```python
from build123d import *

# Parameters (mm, degrees)
F0_R     = 70
F1_DEPTH = 1
F3_R     = 1.99999


# Not quite as in the source:
# - a fillet or chamfer is up to 0.001 mm smaller than in the source, because OpenCascade refuses the exact size
# - a feature of the source that left no trace in its solid (it failed there, or was rolled back) is left out


with BuildPart() as f1:
    # F0 (on Front) → F1 (new body, symmetric)
    with BuildSketch(Plane.XZ):
        Circle(F0_R)
        Polygon((-30.855941539, 30.855941539), (-11.294058461, 42.15), (11.294058461, 42.15), (30.855941539, 30.855941539), (42.15, 11.294058461), (42.15, -11.294058461), (30.855941539, -30.855941539), (11.294058461, -42.15), (-11.294058461, -42.15), (-30.855941539, -30.855941539), (-42.15, -11.294058461), (-42.15, 11.294058461), align=None, mode=Mode.SUBTRACT)
    extrude(amount=F1_DEPTH, both=True)

    # F3 (radius 2 in the source; OpenCascade refuses exactly that, so slightly less here)
    f3_edges = [f1.edges().sort_by_distance(p)[0] for p in [
        (-21.075, -1, 36.502971),
        (0, -1, 42.15),
        (21.075, -1, 36.502971),
        (36.502971, -1, 21.075),
        (42.15, -1, 0),
        (36.502971, -1, -21.075),
        (21.075, -1, -36.502971),
        (0, -1, -42.15),
        (-21.075, -1, -36.502971),
        (-36.502971, -1, -21.075),
        (-42.15, -1, 0),
        (-36.502971, -1, 21.075),
    ]]
    fillet(f3_edges, radius=F3_R)


solid = f1.part
```
Geometry: final body of the model. Coordinates: model frame, mm. Round coordinates to 2 decimals unless told otherwise and drop trailing zeros. Order: outer loops, then holes, each group sorted by start corner. A loop starts at its lowest first (then second) coordinate and runs counter-clockwise, first axis right, second up. Notation, with made-up numbers: (83.25, 32) -> (106.25, 32) arc R7 ccw to (106.25, 42) -> close; hole circle Ø6 at (-27, -18). An arc over 180 degrees is marked (long way). Use one line per item in the form item = value. Start each with the question number.
1. Cut plane C-C (y = -0.5). Return the cut outline in (x, z).
2. Pin query (flat end, axial travel): pin 1 Ø8 at (x, z) = (-31, 29) entering from -Y; pin 2 Ø1 at (y, z) = (0, -44) entering from +X; pin 3 Ø1 at (y, z) = (-0.5, 32) entering from +X. Return the tip coordinate at first contact, or that it passes through.
3. Draft query along X for faces 1 (the face through (-21.23, -0.43, 37.11)), 2 (the face through (-21.52, -0.43, -36.94)), 3 (the face through (30, 1, 32)), 4 (the face through (-55.55, -0.014, -42.594)). Return one class per face: pulls with the +X half, pulls with the -X half, needs draft (parallel to the pull), parting line crosses it, or undercut.
4. Line query: probe 1 along X at (y, z) = (0.3, 3); probe 2 along X at (y, z) = (-0.35, -2.5); probe 3 along Z at (x, y) = (4, -0.15). Output: solid intervals per line, ascending.
5. Cut plane D-D (x = -47). Return the cut outline in (y, z), then the cut area to 4 significant figures.
Solution:
q1.outline = circle Ø140 at (0, 0); hole (-42.83, -11.48) -> (-31.35, -31.35) -> (-11.48, -42.83) -> (11.48, -42.83) -> (31.35, -31.35) -> (42.83, -11.48) -> (42.83, 11.48) -> (31.35, 31.35) -> (11.48, 42.83) -> (-11.48, 42.83) -> (-31.35, 31.35) -> (-42.83, 11.48) -> close
q2.pin_1 = -1
q2.pin_2 = 54.84
q2.pin_3 = 62.51
q3.face_1 = undercut
q3.face_2 = undercut
q3.face_3 = needs draft
q3.face_4 = parting line crosses it
q4.probe_1 = -69.94 to -42.28, 42.28 to 69.94
q4.probe_2 = -69.96 to -42.67, 42.67 to 69.96
q4.probe_3 = -69.89 to -42.51, 42.51 to 69.89
q5.outline = (-1, -51.87) -> (1, -51.87) -> (1, 51.87) -> (-1, 51.87) -> close
q5.area = 207.5 mm^2
